Part model, mm, in its own coordinate system. Face numbers are marked on the shaded views. A direction names the side the tool comes from. Round coordinates to 2 decimals unless told otherwise and drop trailing zeros. Loops run counter-clockwise (first coordinate to the right, second up) from the corner with the lowest first, then second, coordinate; pieces in that order, holes last.
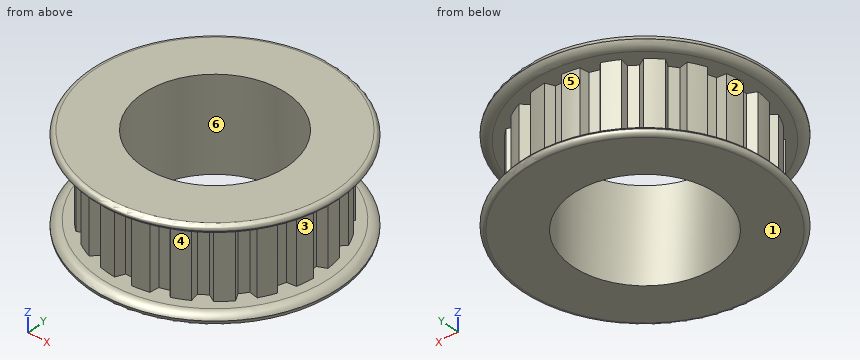
from build123d import *

# Parameters (mm, degrees)
CUT_EXTRUDE1_START     = -9.5
CUT_EXTRUDE1_DEPTH     = 11.2
CIRPATTERN1_COUNT      = 20
SKETCH4_R              = 2
CUT_EXTRUDE2_DEPTH     = 30.034462282
CUT_EXTRUDE3_DEPTH     = 1.5
CIRPATTERN2_COUNT      = 2
CIRPATTERN2_ANGLE      = 90
FILLET1_R              = 0.685714286
FILLET2_R              = 0.24
MOVE_START             = -11
MOVE_FACE1_OUTLINE_R   = 11
MOVE_FACE1_OUTLINE_R_2 = 4
MOVE_FACE1_DEPTH       = 14.2


# Read off the part's stored shape, not the designer's step: Move Face1
with BuildPart() as part:
    # Sketch7 → Revolve1 (revolve)
    with BuildSketch(Plane(origin=(0, 0, 0), x_dir=(0, 0, -1), z_dir=(1, 0, 0)), mode=Mode.PRIVATE) as revolve1_sk:
        with BuildLine():
            Line((-11, 4), (-11, 12))
            Line((-11, 12), (-3.2, 12))
            Line((-3.2, 12), (-3.2, 19))
            Line((-3.2, 19), (-2.45, 19))
            ThreePointArc((-2.45, 19), (-1.899268567, 18.392512657), (-1.7, 17.597127202))
            Line((-1.7, 17.597127202), (-1.7, 16.194254403))
            Line((-1.7, 16.194254403), (9.5, 16.194254403))
            Line((9.5, 16.194254403), (9.5, 17.597127202))
            ThreePointArc((9.5, 17.597127202), (9.699268567, 18.392512657), (10.25, 19))
            Line((10.25, 19), (11, 19))
            Line((11, 19), (11, 4))
            Line((11, 4), (-11, 4))
        make_face()
    revolve(revolve1_sk.sketch.rotate(Axis((0, 0, 11), (0, 0, -1)), 90), axis=Axis((0, 0, 11), (0, 0, -1)))

    # Sketch3 → Cut-Extrude1 (cut)
    with BuildSketch(Plane.XY.offset(CUT_EXTRUDE1_START)):
        with BuildLine():
            Line((-0.690489274, 14.873375), (0.690489274, 14.873375))
            Line((0.690489274, 14.873375), (1.2827, 16.143375))
            ThreePointArc((1.2827, 16.143375), (0, 16.194254403), (-1.2827, 16.143375))
            Line((-1.2827, 16.143375), (-0.690489274, 14.873375))
        make_face()
    cut_extrude1 = extrude(amount=CUT_EXTRUDE1_DEPTH, mode=Mode.SUBTRACT)

    # CirPattern1: Cut-Extrude1 ×20 about axis
    cirpattern1_axis = Axis((0, 0, 0), (0, 0, 1))
    for i in range(1, CIRPATTERN1_COUNT):
        add(cut_extrude1.rotate(cirpattern1_axis, i * 360 / CIRPATTERN1_COUNT), mode=Mode.SUBTRACT)

    # Sketch4 → Cut-Extrude2 (cut, through all)
    with BuildSketch(Plane(origin=(0, 0, 0), x_dir=(1, 0, 0), z_dir=(0, 1, 0))):
        with Locations(Location((0, -7.1, 0), (0, 0, 90))):
            Circle(SKETCH4_R)
    cut_extrude2 = extrude(amount=CUT_EXTRUDE2_DEPTH, mode=Mode.SUBTRACT)

    # Sketch5 → Revolve2 (revolve)
    with BuildSketch(Plane.XY.offset(7.1), mode=Mode.PRIVATE) as revolve2_sk:
        Polygon((0, 11.832159566), (0, 4), (-1.365, 4), (-2, 4.635), (-2, 11.197159566), (-1.365, 11.832159566), align=None)
    revolve2 = revolve(revolve2_sk.sketch.rotate(Axis((0, 0, 7.1), (0, 1, 0)), 270), axis=Axis((0, 0, 7.1), (0, 1, 0)))

    # Sketch6 → Cut-Extrude3 (cut)
    with BuildSketch(Plane(origin=(0, 11.832159566, 0), x_dir=(-1, 0, 0), z_dir=(0, -1, 0))):
        Polygon((0, -5.945299462), (-1, -6.522649731), (-1, -7.677350269), (0, -8.254700538), (1, -7.677350269), (1, -6.522649731), align=None)
    cut_extrude3 = extrude(amount=CUT_EXTRUDE3_DEPTH, mode=Mode.SUBTRACT)

    # CirPattern2: Cut-Extrude2, Revolve2, Cut-Extrude3 ×2 about axis
    cirpattern2_axis = Axis((0, 0, 0), (0, 0, -1))
    add([cut_extrude2.rotate(cirpattern2_axis, i * CIRPATTERN2_ANGLE / (CIRPATTERN2_COUNT - 1)) for i in range(1, CIRPATTERN2_COUNT)], mode=Mode.SUBTRACT)
    add([revolve2.rotate(cirpattern2_axis, i * CIRPATTERN2_ANGLE / (CIRPATTERN2_COUNT - 1)) for i in range(1, CIRPATTERN2_COUNT)])
    add([cut_extrude3.rotate(cirpattern2_axis, i * CIRPATTERN2_ANGLE / (CIRPATTERN2_COUNT - 1)) for i in range(1, CIRPATTERN2_COUNT)], mode=Mode.SUBTRACT)

    # Fillet1
    fillet1_edges = [part.edges().sort_by_distance(p)[0] for p in [
        (-19, 0, -11),
        (-12, 0, 11),
        (-12, 0, 3.2),
        (-19, 0, 3.2),
    ]]
    fillet(fillet1_edges, radius=FILLET1_R)

    # Fillet2
    fillet2_edges = [part.edges().sort_by_distance(p)[0] for p in [
        (-4, 0, -11),
        (-1e-09, 12, 9.100000011),
        (11.832159566, -2, 7.1),
        (-4, 0, 11),
    ]]
    fillet(fillet2_edges, radius=FILLET2_R)

    # Split1
    split(bisect_by=Plane.XY.offset(3.2), keep=Keep.BOTTOM)

    # Move Face1 outline → Move Face1 (cut)
    with BuildSketch(Plane.XY.offset(MOVE_START)):
        Circle(MOVE_FACE1_OUTLINE_R)
        Circle(MOVE_FACE1_OUTLINE_R_2, mode=Mode.SUBTRACT)
    extrude(amount=MOVE_FACE1_DEPTH, mode=Mode.SUBTRACT)


solid = part.part
1) Drop flat-ended pins along their axis: pin 1 Ø10.5 at (x, y) = (0.5, 5) entering from -Z; pin 2 Ø3 at (x, z) = (3.5, -3.5) entering from -Y; pin 3 Ø0.7 at (y, z) = (-0.5, -2.5) entering from -X; pin 4 Ø6 at (y, z) = (-5, -4) entering from +X. Give the stop position or say it passes through.
Values:
pin 1: passes through
pin 2: stops at y = -16.07
pin 3: stops at x = -15.22
pin 4: stops at x = 16.07
2) Mould opens along Y. For the marked faces 4, 5 and 6 say: released by +Y, released by -Y, zero draft, split by the parting line, or undercut.
Values:
face 4: released by -Y
face 5: released by +Y
face 6: undercut
3) Wall check: line 1 along Y through (x, z) = (0, -5.75); line 2 along Y through (x, z) = (-12, 0); line 3 along Z through (x, y) = (-3.5, -16). Give the ranges that are in metal, low to high.
Values:
line 1: y = -14.87 to -11, 11 to 14.87
line 2: y = -10.87 to -9.97, -8.79 to 8.79, 9.97 to 10.87
line 3: z = -11 to -9.5, 1.7 to 3.2
4) Tool access for the marked faces 1, 2 and 3: list every direction of +Z, -Z, +X, -X, +Y, -Y with a clear straight run to the whole face (end or side of a thin tool).
Values:
face 1: -Z, +X, -X, +Y, -Y
face 2: -X, +Y
face 3: +X, -Y
5) Slice it at A-A, the plane y = 0. Give the cut face in (x, z), then the cut area to 3 significant figures.
Values:
outline: (-19, -10.31) arc R0.69 ccw to (-18.31, -11) - (-11, -11) - (-11, 3.2) - (-18.31, 3.2) arc R0.69 ccw to (-19, 2.51) - (-19, 2.45) arc R1.69 ccw to (-17.6, 1.7) - (-14.87, 1.7) - (-14.87, -9.5) - (-17.6, -9.5) arc R1.69 ccw to (-19, -10.25) - close; (11, -11) - (18.31, -11) arc R0.69 ccw to (19, -10.31) - (19, -10.25) arc R1.69 ccw to (17.6, -9.5) - (14.87, -9.5) - (14.87, 1.7) - (17.6, 1.7) arc R1.69 ccw to (19, 2.45) - (19, 2.51) arc R0.69 ccw to (18.31, 3.2) - (11, 3.2) - close
area: 133 mm2
